Autodesk Inventor part; units mm, degrees
ref_plane "YZ Plane" through (0, 0, 0) normal (1, 0, 0) x (0, 1, 0)
ref_plane "XZ Plane" through (0, 0, 0) normal (0, 1, 0) x (-1, 0, 0)
ref_plane "XY Plane" through (0, 0, 0) normal (0, 0, 1) x (1, 0, 0)
sketch "Sketch9" plane through (0, 0, 0) normal (0, 0, 1) x (1, 0, 0)
  line L0 (0, 0) -> (395.8194, 0)
  line L1 (387.9689, -2.54) -> (508, -123.4756)
  line L2 (508, -123.4756) -> (508, -228.3729)
  line L3 (517.1565, -218.6006) -> (386.5644, -411.48)
  line L4 (386.5644, -411.48) -> (0, -411.48)
  line L5 (0, -411.48) -> (0, -408.94)
  line L6 (0, -408.94) -> (385.7441, -408.94)
  line L7 (385.7441, -408.94) -> (508, -228.3729)
  line L8 (517.1565, -218.6006) -> (517.1565, -122.2514)
  line L9 (517.1565, -122.2514) -> (395.8194, 0)
  line L10 (387.9689, -2.54) -> (0, -2.54)
  line L11 (0, -2.54) -> (0, 0)
  dimension "d32" = 508
  dimension "d35" = 406.4
  dimension "d36" = 2.54
  dimension "d37" = 2.54
extrude "Extrusion6" add sketch "Sketch9" along normal blind 25.4
hole "Hole1" at (12.7, 0, 12.7) direction (0, -1, 0) diameter 12.7 end through all
hole "Hole2" at (203.2, 0, 12.7) direction (0, -1, 0) diameter 12.7 end through all
properties part number "4barRoundedBar"
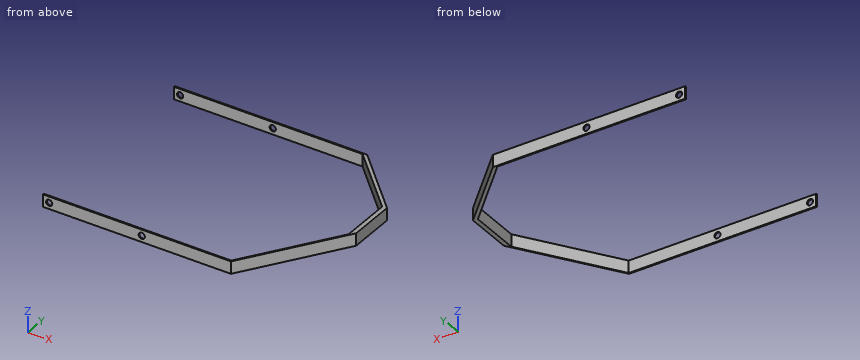
Geometry: final body of the model. Coordinates: model frame, mm. Round coordinates to 2 decimals unless told otherwise and drop trailing zeros. Order: outer loops, then holes, each group sorted by start corner. A loop starts at its lowest first (then second) coordinate and runs counter-clockwise, first axis right, second up. Notation, with made-up numbers: M -9.75,34 L 42.25,34 A26 ccw 42.25,50 Z; hole C 45.25,56.5 d11. An arc over 180 degrees is marked long. One line per item, written item: value.
(1) Cut plane B-B (z = 12.7). Return the cut outline in (x, y).
Result sheet:
outline: M 0,-411.48 L 6.35,-411.48 L 6.35,-408.94 L 0,-408.94 Z; M 0,-2.54 L 6.35,-2.54 L 6.35,0 L 0,0 Z; M 19.05,-411.48 L 196.85,-411.48 L 196.85,-408.94 L 19.05,-408.94 Z; M 19.05,-2.54 L 196.85,-2.54 L 196.85,0 L 19.05,0 Z; M 209.55,-411.48 L 386.56,-411.48 L 517.16,-218.6 L 517.16,-122.25 L 395.82,0 L 209.55,0 L 209.55,-2.54 L 387.97,-2.54 L 508,-123.48 L 508,-228.37 L 385.74,-408.94 L 209.55,-408.94 Z
(2) Line query: probe 1 along X at (y, z) = (-409.45, 12.7); probe 2 along Z at (x, y) = (12.7, -409.7); probe 3 along Y at (x, z) = (185.5, 19.25). Output: solid intervals per line, ascending. Write a range as [from, to].
Result sheet:
probe 1: [0, 6.35], [19.05, 196.85], [209.55, 387.94]
probe 2: [0, 6.35], [19.05, 25.4]
probe 3: [-411.48, -408.94], [-2.54, 0]
(3) Cut plane A-A (x = 203.2). Return the cut outline in (y, z), and give its area (3 significant figures).
Result sheet:
outline: M -411.48,0 L -408.94,0 L -408.94,6.35 L -411.48,6.35 Z; M -411.48,19.05 L -408.94,19.05 L -408.94,25.4 L -411.48,25.4 Z; M -2.54,0 L 0,0 L 0,6.35 L -2.54,6.35 Z; M -2.54,19.05 L 0,19.05 L 0,25.4 L -2.54,25.4 Z
area: 64.5 mm2
(4) Cut plane D-D (y = -184.5). Return the cut outline in (x, z).
Result sheet:
outline: M 508,0 L 517.16,0 L 517.16,25.4 L 508,25.4 Z
(5) Pin query (flat end, axial travel): P1, Ø11.5, axis at x = 203.2, z = 12.7, coming from the -Y side; P2, Ø10, axis at x = 457.5, z = 7.5, coming from the -Y side; P3, Ø4, axis at x = 453, z = 15, coming from the +Y side. Return the tip coordinate at first contact, or that it passes through.
Result sheet:
P1: through
P2: y = -314.1
P3: y = -55.6
(6) Cut plane C-C (x = 133). Return the cut outline in (y, z), and give its area (3 significant figures).
Result sheet:
outline: M -411.48,0 L -408.94,0 L -408.94,25.4 L -411.48,25.4 Z; M -2.54,0 L 0,0 L 0,25.4 L -2.54,25.4 Z
area: 129 mm2
